```python
from build123d import *

# Parameters (mm, degrees)
F1_DEPTH = 1
F2_DEPTH = 6
F5_DEPTH = 25
F8_DEPTH = 19.4554531584


with BuildPart() as f1:
    # F0 (on Top) → F1 (new body)
    with BuildSketch(Plane.XY):
        Polygon((-29.4488155034, 5.7242698613), (0, 0), (29.4488155034, 5.7242698613), (28.8382267182, 8.8654768483), (0, 3.2598934239), (-28.8382267182, 8.8654768483), align=None)
        Polygon((29.4488155034, 5.7242698613), (0, 0), (-29.4488155034, 5.7242698613), (-29.5633009007, 5.1352935512), (0, -0.611230017), (29.5633009007, 5.1352935512), align=None)
        Polygon((0, 3.2598934239), (28.8382267182, 8.8654768483), (28.723741321, 9.4544531584), (0, 3.8711234408), (-28.723741321, 9.4544531584), (-28.8382267182, 8.8654768483), align=None)
    extrude(amount=-F1_DEPTH)

    # F0 (on Top) → F2 (join)
    with BuildSketch(Plane.XY):
        Polygon((0, 3.2598934239), (28.8382267182, 8.8654768483), (28.723741321, 9.4544531584), (0, 3.8711234408), (-28.723741321, 9.4544531584), (-28.8382267182, 8.8654768483), align=None)
        Polygon((29.4488155034, 5.7242698613), (0, 0), (-29.4488155034, 5.7242698613), (-29.5633009007, 5.1352935512), (0, -0.611230017), (29.5633009007, 5.1352935512), align=None)
    extrude(amount=F2_DEPTH)

    # F4 (on face) → F5 (cut)
    with BuildSketch(Plane(origin=(0.7250741824, 3.7301832971, 0), x_dir=(-0.9816271834, 0.1908089954, 0), z_dir=(0.1908089954, 0.9816271834, 0))):
        Polygon((30, 2), (30, 6), (8.7386451747, 6), align=None)
    extrude(amount=-F5_DEPTH, mode=Mode.SUBTRACT)

    # F7 (on offset) → F8 (cut, through all)
    with BuildSketch(Plane.XZ.offset(10)):
        Polygon((-30.2472151816, -2.2539433558), (0, -2.2539433558), (0, -1), (0, 10.581173934), (-30.2472151816, 10.581173934), align=None)
        Polygon((0, 10.581173934), (0, -1), (1.0596845285, 11.1122495846), align=None)
    extrude(amount=-F8_DEPTH, mode=Mode.SUBTRACT)

    # F10: F1 across plane


with BuildPart() as f1_1:
    add(f1.part)
    add(f1.part.mirror(Plane(origin=(0.2338059111, 1.6753939772, 1.6724137931), x_dir=(0, -1, 0), z_dir=(-0.9961946981, 0, 0.0871557427))))


solid = f1_1.part
```
The listing builds one solid part. Answer for the finished solid, in the listing's coordinates (mm). A direction names the side the tool comes from. Coordinates: 2 decimals unless noted, no trailing zeros. Write each loop counter-clockwise with the first axis right and the second up, starting at its lowest first coordinate (ties: lowest second). Pieces come first, ordered by that corner, then holes. Notation, with made-up numbers: (43, 21.5) - (74, 21.5) arc R27 ccw to (74, 47.5) - close; hole circle Ø1 at (22.25, 60.5). An arc over 180 degrees is marked (long way). One line per item, written item: value.
1) Consider line 1 along Y through (x, z) = (-8, 2.75); line 2 along Z through (x, y) = (22, 7.5); line 3 along Z through (x, y) = (18.5, 3.5). Determine where each line is inside the solid, lowest interval first. Write a range as from..to.
Geometry check:
line 1: y = 1.05..1.66, 4.92..5.53
line 2: z = -1..0
line 3: z = -1..6
2) Find section B-B (y = 7.75). Give the vertices of the cut face in (x, z).
Geometry check:
outline: (-28.61, 4.05) - (-19.65, 2.47) - (-18.44, 9.36) - (-21.53, 9.9) - (-22.58, 4) - (-28.44, 5.03) - close; (19.96, -1) - (29.06, -1) - (29.06, 0) - (23.1, 0) - (23.1, 6) - (19.96, 6) - close
3) Find section A-A (z = 9.75). Give the vertices of the cut face in (x, y), and give its area (3 significant figures).
Geometry check:
outline: (-28.12, 5.14) - (-20.65, 3.71) - (-20.65, 4.32) - (-28.01, 5.72) - close; (-27.39, 8.87) - (-20.65, 7.58) - (-20.65, 8.19) - (-27.27, 9.45) - close
area: 8.61 mm2
4) Find section D-D (z = 3). Give the vertices of the cut face in (x, y), and give its area (3 significant figures).
Geometry check:
outline: (-22.69, 3.87) - (0.35, -0.54) - (29.56, 5.14) - (29.45, 5.72) - (0.35, 0.07) - (-16.93, 3.38) - (-16.93, 6.64) - (0.35, 3.33) - (28.84, 8.87) - (28.72, 9.45) - (0.35, 3.94) - (-22.69, 8.35) - close
area: 82.1 mm2
5) A tool of negligible diameter and unlimited length cuts with its end or side. For faces 4 (the flat face through (14.26, 6.03, 2.96)), 5 (the flat face through (15, 2.6, 6)), 6 (the flat face through (14.57, 2.22, 2.55)), from which of +Z, -Z, +X, -X, +Y, -Y can it reach the whole face along a straight path? Write none if from no direction.
Geometry check:
face 4: +Z
face 5: +Z, +X, +Y, -Y
face 6: +Z, -Z, +X, -Y
6) For a pull along X with two mould halves and no side action, classify faces 1 (the flat face through (-14.35, 4.49, 1.53)), 2 (the flat face through (15, 4, -1)), 3 (the flat face through (-14.168, 4.503, 2.514)) as pulls with the +X half, pulls with the -X half, needs draft (parallel to the pull), parting line crosses it, or undercut.
Geometry check:
face 1: pulls with the -X half
face 2: needs draft
face 3: undercut
7) Each of these flat-tipped pins is pushed along its axis until it touches: pin 1 Ø1 at (x, z) = (16, 0.5) entering from +Y; pin 2 Ø4 at (x, y) = (-13.5, 2.5) entering from +Z; pin 3 Ø5 at (x, y) = (8, 5) entering from +Z. Where does it stop, or does it pass through?
Geometry check:
pin 1: stops at y = 7.08
pin 2: stops at z = 8.84
pin 3: stops at z = 6
8) Find section C-C (x = 10). Give the vertices of the cut face in (y, z).
Geometry check:
outline: (1.33, -1) - (5.81, -1) - (5.81, 6) - (5.2, 6) - (5.2, 0) - (1.94, 0) - (1.94, 6) - (1.33, 6) - close
